```python
from build123d import *

# Parameters (mm, degrees)
SKETCH3_R          = 30.175
CUT_EXTRUDE1_DEPTH = 59.15
CHAMFER1_SIZE      = 0.75
CHAMFER2_SIZE      = 3
CHAMFER2_SIZE2     = 5.196152423
FILLET1_R          = 3


with BuildPart() as part:
    # Sketch2 → Revolve1 (revolve)
    with BuildSketch(Plane.XY):
        Polygon((0, 0), (0, 58.15), (-35, 58.15), (-35, 7.35), (-41.35, 7.35), (-41.35, 1), (-31.75, 1), (-31.75, 0), align=None)
    revolve(axis=Axis((0, 0, 0), (0, 1, 0)))

    # Sketch3 → Cut-Extrude1 (cut, through all)
    with BuildSketch(Plane(origin=(0, 58.15, 0), x_dir=(1, 0, 0), z_dir=(0, 1, 0))):
        Circle(SKETCH3_R)
    extrude(amount=-CUT_EXTRUDE1_DEPTH, mode=Mode.SUBTRACT)

    # Chamfer1
    chamfer1_edges = [part.edges().sort_by_distance(p)[0] for p in [
        (35, 7.35, 0),
        (35, 58.15, 0),
    ]]
    chamfer(chamfer1_edges, length=CHAMFER1_SIZE)

    # Chamfer2
    chamfer2_edges = [part.edges().sort_by_distance(p)[0] for p in [
        (41.35, 7.35, 0),
    ]]
    chamfer2_side = [part.faces().sort_by_distance(p)[0] for p in [
        (41.35, 4.175, 0),
    ]]
    chamfer(chamfer2_edges, length=CHAMFER2_SIZE, length2=CHAMFER2_SIZE2, reference=chamfer2_side[0])

    # Fillet1
    fillet1_edges = [part.edges().sort_by_distance(p)[0] for p in [
        (-30.175, 58.15, 0),
    ]]
    fillet(fillet1_edges, radius=FILLET1_R)


solid = part.part
```
Can you work these out from the model? Positions are in its coordinate system, mm. A direction names the side the tool comes from. Coordinates: 2 decimals unless noted, no trailing zeros. Loops run counter-clockwise (first coordinate to the right, second up) from the corner with the lowest first, then second, coordinate; pieces in that order, holes last. Notation, with made-up numbers: (57.25, 24.25) - (74.25, 24.25) arc R30 ccw to (74.25, 59.25) - close; hole circle Ø8 at (78.5, 34). An arc over 180 degrees is marked (long way). Answer as CSV lines item,"result". Start each with the question number.
1) Thinking about a two-plate mould opening in X: for faces 1 (the conical face through (28.891, 7.204, -22.153)), 2 (the flat face through (-28, 0, -12)), 3 (the cylindrical face through (-23.946, 27.961, 18.361)), which applies, pulls with the +X half, pulls with the -X half, needs draft (parallel to the pull), parting line crosses it, or undercut?
2) Suppose I cut it at B-B (z = 0). Please give me the cut outline in (x, y) (3 decimals).
3) For pin 1 (4 mm diameter, centred on y = 11, z = -0.5, fed in from +X); pin 2 (8 mm diameter, centred on y = 11, z = -23, fed in from -X); pin 3 (2 mm diameter, centred on y = 31, z = -2.5, fed in from -X), each with a flat end and sliding along its axis, tell me the tip position at first contact or that it passes through.
4) I need wall thicknesses on line 1 (Z direction, x = 0, y = 42) (3 decimals); line 2 (X direction, y = 9.5, z = 15.5); line 3 (X direction, y = 39, z = 16.5). Which ranges of each line are inside material? Lowest first, please. Write a range as from..to.
5) Which directions (+Z, -Z, +X, -X, +Y, -Y) give clear straight access to the entire face, cutting with the end or side of a thin tool? Please do faces 4 (the cylindrical face through (8.964, 2.652, -40.367)), 5 (the cylindrical face through (28, 32, -21)), 6 (the flat face through (-12, 1, -30)).
6) Suppose I cut it at A-A (x = 0). Please give me the cut outline in (y, z) (3 decimals).
7) Suppose I cut it at C-C (y = 43). Please give me the cut outline in (x, z) (3 decimals), plus the area to 3 significant figures.
Check result:
1,face 1,"parting line crosses it"
1,face 2,"needs draft"
1,face 3,"undercut"
2,outline,"(-41.35, 1) - (-31.75, 1) - (-31.75, 0) - (-30.175, 0) - (-30.175, 55.15) arc R3 ccw to (-33.175, 58.15) - (-34.25, 58.15) - (-35, 57.4) - (-35, 8.1) - (-35.75, 7.35) - (-36.154, 7.35) - (-41.35, 4.35) - close; (30.175, 0) - (31.75, 0) - (31.75, 1) - (41.35, 1) - (41.35, 4.35) - (36.154, 7.35) - (35.75, 7.35) - (35, 8.1) - (35, 57.4) - (34.25, 58.15) - (33.175, 58.15) arc R3 ccw to (30.175, 55.15) - close"
3,pin 1,"stops at x = 35"
3,pin 2,"stops at x = -29.39"
3,pin 3,"stops at x = -34.97"
4,line 1,"z = -35..-30.175, 30.175..35"
4,line 2,"x = -31.38..-25.89, 25.89..31.38"
4,line 3,"x = -30.87..-25.26, 25.26..30.87"
5,face 4,"+Y, -Y"
5,face 5,"+Y"
5,face 6,"-Y"
6,outline,"(0, -31.75) - (1, -31.75) - (1, -41.35) - (4.35, -41.35) - (7.35, -36.154) - (7.35, -35.75) - (8.1, -35) - (57.4, -35) - (58.15, -34.25) - (58.15, -33.175) arc R3 ccw to (55.15, -30.175) - (0, -30.175) - close; (0, 30.175) - (55.15, 30.175) arc R3 ccw to (58.15, 33.175) - (58.15, 34.25) - (57.4, 35) - (8.1, 35) - (7.35, 35.75) - (7.35, 36.154) - (4.35, 41.35) - (1, 41.35) - (1, 31.75) - (0, 31.75) - close"
7,outline,"circle Ø70 at (0, 0); hole circle Ø60.35 at (0, 0)"
7,area,"988 mm²"
